The listing builds one solid part. Answer for the finished solid, in the listing's coordinates (mm). Coordinates: 2 decimals unless noted, no trailing zeros.
from build123d import *

# Parameters (mm, degrees)
SKETCH1_W           = 952.5
SKETCH1_H           = 190.5
BOSS_EXTRUDE1_DEPTH = 12.7
SKETCH5_W           = 127
SKETCH5_H           = 38.1
CUT_EXTRUDE3_DEPTH  = 486.84762529
FILLET1_R           = 12.7
SKETCH6_R           = 3.175
CUT_EXTRUDE4_DEPTH  = 11.43
SKETCH7_R           = 2.5
CUT_EXTRUDE5_DEPTH  = 8
SKETCH8_R           = 2.5
CUT_EXTRUDE6_DEPTH  = 8
SKETCH9_R           = 3.175
CUT_EXTRUDE7_DEPTH  = 11.43


with BuildPart() as part:
    # Sketch1 → Boss-Extrude1 (new body)
    with BuildSketch(Plane.XY):
        Rectangle(SKETCH1_W, SKETCH1_H)
    extrude(amount=BOSS_EXTRUDE1_DEPTH)

    # Sketch5 → Cut-Extrude3 (cut, through all)
    with BuildSketch(Plane.XY.offset(12.7)):
        with Locations((3.078763255, 76.2)):
            Rectangle(SKETCH5_W, SKETCH5_H)
    extrude(amount=-CUT_EXTRUDE3_DEPTH, mode=Mode.SUBTRACT)

    # Fillet1
    fillet1_edges = [part.edges().sort_by_distance(p)[0] for p in [
        (66.578763255, 95.25, 6.35),
        (66.578763255, 57.15, 6.35),
        (-60.421236745, 57.15, 6.35),
        (-60.421236745, 95.25, 6.35),
    ]]
    fillet(fillet1_edges, radius=FILLET1_R)

    # Sketch6 → Cut-Extrude4 (cut)
    with BuildSketch(Plane(origin=(0, 0, 0), x_dir=(-1, 0, 0), z_dir=(0, 0, -1))):
        with Locations((-425.45, 0)):
            Circle(SKETCH6_R)
        with Locations(Location((425.45, 0, 0), (0, 0, 180))):
            Circle(SKETCH6_R)
    extrude(amount=-CUT_EXTRUDE4_DEPTH, mode=Mode.SUBTRACT)

    # Sketch7 → Cut-Extrude5 (cut)
    with BuildSketch(Plane(origin=(0, 0, 0), x_dir=(-1, 0, 0), z_dir=(0, 0, -1))):
        with Locations((-425.45, 44.45)):
            Circle(SKETCH7_R)
        with Locations(Location((-425.45, -44.45, 0), (0, 0, 180))):
            Circle(SKETCH7_R)
        with Locations((425.45, -44.45)):
            Circle(SKETCH7_R)
        with Locations(Location((425.45, 44.45, 0), (0, 0, 180))):
            Circle(SKETCH7_R)
    extrude(amount=-CUT_EXTRUDE5_DEPTH, mode=Mode.SUBTRACT)

    # Sketch8 → Cut-Extrude6 (cut)
    with BuildSketch(Plane(origin=(0, 0, 0), x_dir=(-1, 0, 0), z_dir=(0, 0, -1))):
        with Locations((-425.45, -82.55)):
            Circle(SKETCH8_R)
        with Locations((-212.725, -82.55)):
            Circle(SKETCH8_R)
        with Locations((0, -82.55)):
            Circle(SKETCH8_R)
        with Locations((212.725, -82.55)):
            Circle(SKETCH8_R)
        with Locations((425.45, -82.55)):
            Circle(SKETCH8_R)
    extrude(amount=-CUT_EXTRUDE6_DEPTH, mode=Mode.SUBTRACT)

    # Sketch9 → Cut-Extrude7 (cut)
    with BuildSketch(Plane(origin=(0, 0, 0), x_dir=(-1, 0, 0), z_dir=(0, 0, -1))):
        with Locations((-319.0875, -82.55)):
            Circle(SKETCH9_R)
        with Locations((-106.3625, -82.55)):
            Circle(SKETCH9_R)
        with Locations((106.3625, -82.55)):
            Circle(SKETCH9_R)
        with Locations((319.0875, -82.55)):
            Circle(SKETCH9_R)
    extrude(amount=-CUT_EXTRUDE7_DEPTH, mode=Mode.SUBTRACT)


solid = part.part
Q1. The part is cut by section A-A, the plane z = 6. State how many separate pieces and enclosed holes the cut face has, then the cut area to 3 significant figures.
Answers below:
separate pieces: 1
enclosed holes: 15
area: 176,000 mm2
Q2. Find the intervals of material crossed by probe 1 along Y at (x, z) = (425.45, 4) (3 decimals); probe 2 along Y at (x, z) = (0, 5.25); probe 3 along X at (y, z) = (2.5, 0.5), in increasing order.
Answers below:
probe 1: y = -95.25 to -85.05, -80.05 to -46.95, -41.95 to -3.175, 3.175 to 41.95, 46.95 to 95.25
probe 2: y = -95.25 to -85.05, -80.05 to 57.15
probe 3: x = -476.25 to -427.41, -423.49 to 423.49, 427.41 to 476.25
Q3. Given pin 1 (1.9 mm diameter, centred on x = -107.5, y = -81.5, fed in from -Z); pin 2 (1.5 mm diameter, centred on x = -426.5, y = 44, fed in from -Z), each flat-ended and moving along its own axis, determine where each tip first touches the part or whether it passes through.
Answers below:
pin 1: stops at z = 11.43
pin 2: stops at z = 8
